```python
from build123d import *

# Parameters (mm, degrees)
PAD062_DEPTH    = 30
SKETCH125_W     = 10
SKETCH125_H     = 13
POCKET062_DEPTH = 4
SKETCH126_W     = 60
SKETCH126_H     = 5
PAD063_DEPTH    = 3
SKETCH127_W     = 13
SKETCH127_H     = 17
PAD064_DEPTH    = 3
SKETCH128_W     = 3
SKETCH128_H     = 12
PAD065_DEPTH    = 10
SKETCH129_R     = 1.7
POCKET063_DEPTH = 5
CHAMFER046_SIZE = 3
FILLET045_R     = 3
FILLET046_R     = 3
CHAMFER047_SIZE = 1
SKETCH130_R     = 2.15
POCKET064_DEPTH = 10.001
CHAMFER048_SIZE = 0.4


with BuildPart() as part:
    # Sketch124 → Pad062 (new body, symmetric)
    with BuildSketch(Plane.YZ):
        Polygon((-10, 0), (-10, 10), (0, 10), (0, 0), (0, -3), (0, -8), (-10, -8), (-10, -3), (-1, -3), (-1, 0), align=None)
    extrude(amount=PAD062_DEPTH, both=True)

    # Sketch125 (on Face8 of Pad062) → Pocket062 (cut)
    with BuildSketch(Plane(origin=(-30, 0, 0), x_dir=(0, -1, 0), z_dir=(-1, 0, 0))):
        with Locations((5, 3.5)):
            Rectangle(SKETCH125_W, SKETCH125_H)
    pocket062 = extrude(amount=-POCKET062_DEPTH, mode=Mode.SUBTRACT)

    # Mirrored009: Pocket062 across YZ
    add(pocket062.mirror(Plane.YZ), mode=Mode.SUBTRACT)

    # Sketch126 (on Face6 of Mirrored009) → Pad063 (join)
    with BuildSketch(Plane(origin=(0, 0, 0), x_dir=(-1, 0, 0), z_dir=(0, 1, 0))):
        with Locations((0, -5.5)):
            Rectangle(SKETCH126_W, SKETCH126_H)
    extrude(amount=PAD063_DEPTH)

    # Sketch127 → Pad064 (join)
    with BuildSketch(Plane.XZ):
        with Locations((33.5, 0.5)):
            Rectangle(SKETCH127_W, SKETCH127_H)
    pad064 = extrude(amount=-PAD064_DEPTH)

    # Sketch128 (on Face6 of Pad064) → Pad065 (join)
    with BuildSketch(Plane.XZ):
        with Locations((28.5, 3)):
            Rectangle(SKETCH128_W, SKETCH128_H)
    pad065 = extrude(amount=PAD065_DEPTH)

    # Mirrored010: Pad064, Pad065 across Sketch127 V_Axis
    add(pad064.mirror(Plane(origin=(0, 0, 0), x_dir=(0, -1, 0), z_dir=(1, 0, 0))))
    add(pad065.mirror(Plane(origin=(0, 0, 0), x_dir=(0, -1, 0), z_dir=(1, 0, 0))))

    # Sketch129 → Pocket063 (cut)
    with BuildSketch(Plane.XZ):
        with Locations((-35, 0.5)):
            Circle(SKETCH129_R)
        with Locations((35, 0.5)):
            Circle(SKETCH129_R)
    extrude(amount=-POCKET063_DEPTH, mode=Mode.SUBTRACT)

    # Chamfer046
    chamfer046_edges = [part.edges().sort_by_distance(p)[0] for p in [
        (-40, 1.5, 9),
        (-40, 1.5, -8),
        (40, 1.5, -8),
        (40, 1.5, 9),
    ]]
    chamfer(chamfer046_edges, length=CHAMFER046_SIZE)

    # Fillet045
    fillet045_edges = [part.edges().sort_by_distance(p)[0] for p in [
        (-30, -5, -8),
        (30, -5, -8),
    ]]
    fillet(fillet045_edges, radius=FILLET045_R)

    # Fillet046
    fillet046_edges = [part.edges().sort_by_distance(p)[0] for p in [
        (26, -5.5, 0),
        (-26, -5.5, 0),
    ]]
    fillet(fillet046_edges, radius=FILLET046_R)

    # Chamfer047
    chamfer047_edges = [part.edges().sort_by_distance(p)[0] for p in [
        (-28.5, -10, 9),
        (28.5, -10, 9),
        (0, -10, 10),
    ]]
    chamfer(chamfer047_edges, length=CHAMFER047_SIZE)

    # Sketch130 (on Face7 of Chamfer047) → Pocket064 (cut, through all)
    with BuildSketch(Plane(origin=(0, 0, 0), x_dir=(-1, 0, 0), z_dir=(0, 1, 0))):
        with Locations((-20, 5)):
            Circle(SKETCH130_R)
        with Locations((20, 5)):
            Circle(SKETCH130_R)
    extrude(amount=-POCKET064_DEPTH, mode=Mode.SUBTRACT)

    # Chamfer048
    chamfer048_edges = [part.edges().sort_by_distance(p)[0] for p in [
        (-17.85, -10, 5),
        (-17.85, 0, 5),
        (22.15, -10, 5),
        (22.15, 0, 5),
    ]]
    chamfer(chamfer048_edges, length=CHAMFER048_SIZE)


solid = part.part
```
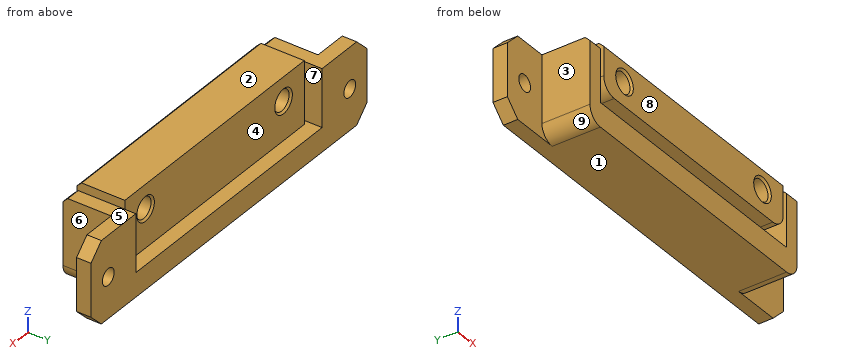
Can you work these out from the model? Positions are in its coordinate system, mm. Face numbers are marked on the shaded views. A direction names the side the tool comes from. Give positions to 0.01 mm unless a question says otherwise; leave off trailing zeros. Loops run counter-clockwise (first coordinate to the right, second up) from the corner with the lowest first, then second, coordinate; pieces in that order, holes last. Notation, with made-up numbers: M 58,20.5 L 64,20.5 A24 ccw 64,59.5 Z; hole C -29.75,9.5 d7. An arc over 180 degrees is marked long. Use one line per item in the form item = value. Start each with the question number.
(1) On a 3-axis mill with a long thin cutter (end or side, diameter ignored), from which of +Z, -Z, +X, -X, +Y, -Y can I reach the whole of each face in a straight line? I mean the marked faces 1, 2, 3, 4 and 5. Say none if no direction works.
(2) I want a section at D-D, the plane x = 3.5. Write out the boundary of the cut face in (y, z), and give its area (4 significant figures).
(3) Thinking about a two-plate mould opening in X: for the marked faces 6, 7, 8 and 9, which applies, released by +X, released by -X, zero draft, split by the parting line, or undercut?
(4) I want a section at C-C, the plane z = 5. State how many separate pieces and enclosed holes the cut face has, and give its area (3 significant figures).
(5) I want a section at A-A, the plane x = -20. Write out the boundary of the cut face in (y, z).
(6) I'm going to push flat-ended pins straight in: P1, Ø2, axis at x = 35, z = 0.5, coming from the -Y side; P2, Ø5, axis at y = -6.5, z = 1, coming from the -X side; P3, Ø10.5, axis at x = 1.5, z = 2.5, coming from the +Y side; P4, Ø10.5, axis at x = -34.5, z = 3, coming from the -Y side. Where does each tip first touch, or does it pass through?
(7) I want a section at B-B, the plane y = 1.5. Write out the boundary of the cut face in (x, z), and give its area (3 significant figures).
Worked out:
q1.face_1 = -Z, +X, -X, +Y, -Y
q1.face_2 = +Z, +X, -X, +Y, -Y
q1.face_3 = +Z, -Z, -X, -Y
q1.face_4 = +Z, +Y
q1.face_5 = +Z, +X, +Y, -Y
q2.outline = M -10,-8 L 3,-8 L 3,-3 L 0,-3 L 0,10 L -9,10 L -10,9 L -10,0 L -1,0 L -1,-3 L -10,-3 Z
q2.area = 167.5 mm²
q3.face_6 = released by +X
q3.face_7 = undercut
q3.face_8 = zero draft
q3.face_9 = released by -X
q4.separate_pieces = 5
q4.enclosed_holes = 0
q4.area = 571 mm²
q5.outline = M -10,-8 L 3,-8 L 3,-3 L 0,-3 L 0,2.45 L -0.4,2.85 L -9.6,2.85 L -10,2.45 L -10,0 L -1,0 L -1,-3 L -10,-3 Z; M -10,7.55 L -9.6,7.15 L -0.4,7.15 L 0,7.55 L 0,10 L -9,10 L -10,9 Z
q6.P1 = through
q6.P2 = -30
q6.P3 = 0
q6.P4 = -10
q7.outline = M -40,-5 L -37,-8 L 37,-8 L 40,-5 L 40,6 L 37,9 L 27,9 L 27,-3 L -27,-3 L -27,9 L -37,9 L -40,6 Z; hole C -35,0.5 d3.4; hole C 35,0.5 d3.4
q7.area = 676 mm²
